Work out the finished part from the listing and answer in its coordinate system (mm). A direction names the side the tool comes from. Round coordinates to 2 decimals unless told otherwise and drop trailing zeros. Order: outer loops, then holes, each group sorted by start corner. A loop starts at its lowest first (then second) coordinate and runs counter-clockwise, first axis right, second up. Notation, with made-up numbers: M 14,-5.5 L 56,-5.5 A7 ccw 56,3.5 Z; hole C 19.5,74 d10. An arc over 180 degrees is marked long. Return JSON: item names as keys, results as strings.
from build123d import *

# Parameters (mm, degrees)
SKETCH1_W             = 66.04
SKETCH1_H             = 33.02
BOSS_EXTRUDE1_DEPTH   = 4.2418
FILLET1_R             = 1.27
SKETCH2_W             = 106.172
SKETCH2_H             = 36.322
BOSS_EXTRUDE2_DEPTH   = 6.604
F_3_CLEARANCE_HOLE1_D = 2.794
SKETCH6_W             = 69.85
SKETCH6_H             = 22.606
BOSS_EXTRUDE3_DEPTH   = 22.0472


with BuildPart() as part:
    # Sketch1 → Boss-Extrude1 (new body)
    with BuildSketch(Plane(origin=(0, 0, 0), x_dir=(1, 0, 0), z_dir=(0, 1, 0))):
        Rectangle(SKETCH1_W, SKETCH1_H)
    extrude(amount=BOSS_EXTRUDE1_DEPTH)

    # Fillet1
    fillet1_edges = [part.edges().sort_by_distance(p)[0] for p in [
        (33.02, 2.1209, 16.51),
        (-33.02, 2.1209, 16.51),
        (-33.02, 2.1209, -16.51),
        (33.02, 2.1209, -16.51),
    ]]
    fillet(fillet1_edges, radius=FILLET1_R)

    # Sketch2 → Boss-Extrude2 (add)
    with BuildSketch(Plane.XZ):
        Rectangle(SKETCH2_W, SKETCH2_H)
    extrude(amount=BOSS_EXTRUDE2_DEPTH)

    # #3 Clearance Hole1 (through all)
    with Locations(Plane(origin=(0, 0, 0), x_dir=(1, 0, 0), z_dir=(0, 1, 0))):
        with Locations((-48.3997, 0), (48.3997, 0)):
            Hole(F_3_CLEARANCE_HOLE1_D / 2)

    # Sketch6 → Boss-Extrude3 (add)
    with BuildSketch(Plane.XZ.offset(6.604)):
        Rectangle(SKETCH6_W, SKETCH6_H)
    extrude(amount=BOSS_EXTRUDE3_DEPTH)


solid = part.part
Item 1: Which of the six approach directions +Z, -Z, +X, -X, +Y, -Y give full straight-line access (tool end or side, diameter ignored) to faces 1 (the flat face through (-34.925, -17, 0)), 2 (the flat face through (-33.02, 2, 0)), 3 (the flat face through (33.02, 2, 0)), 4 (the flat face through (0, 2, 16.51)), 5 (the flat face through (0, -17, 11.303))?
Output:
{"face 1": "+Z, -Z, -X, -Y", "face 2": "+Z, -Z, -X, +Y", "face 3": "+Z, -Z, +X, +Y", "face 4": "+Z, +X, -X, +Y", "face 5": "+Z, +X, -X, -Y"}
Item 2: Find section C-C (y = -17.5). Determine the outline of the cut face in (x, z) (3 decimals).
Output:
{"outline": "M -34.925,-11.303 L 34.925,-11.303 L 34.925,11.303 L -34.925,11.303 Z"}
Item 3: Each of these flat-tipped pins is pushed along its axis until it touches: pin 1 (2.5 mm diameter, centred on x = 48.4, z = 0, fed in from +Y); pin 2 (11 mm diameter, centred on y = -20, z = 3, fed in from -X) (3 decimals); pin 3 (4 mm diameter, centred on x = 4, y = -24, fed in from -Z); pin 4 (1.3 mm diameter, centred on y = 2.5, z = -6.5, fed in from +X). Where does it stop, or does it pass through?
Output:
{"pin 1": "passes through", "pin 2": "stops at x = -34.925", "pin 3": "stops at z = -11.3", "pin 4": "stops at x = 33.02"}
Item 4: Consider line 1 along Z through (x, y) = (11, -22.5); line 2 along Y through (x, z) = (26, -12); line 3 along X through (y, z) = (-21, 9) (3 decimals). Determine where each line is inside the solid, lowest interval first. Write a range as [from, to].
Output:
{"line 1": "z = [-11.3, 11.3]", "line 2": "y = [-6.6, 4.24]", "line 3": "x = [-34.925, 34.925]"}
Item 5: Find section D-D (z = -9). Determine the outline of the cut face in (x, y) (3 decimals).
Output:
{"outline": "M -53.086,-6.604 L -34.925,-6.604 L -34.925,-28.651 L 34.925,-28.651 L 34.925,-6.604 L 53.086,-6.604 L 53.086,0 L 33.02,0 L 33.02,4.242 L -33.02,4.242 L -33.02,0 L -53.086,0 Z"}
Item 6: Find section A-A (z = 0). Determine the outline of the cut face in (x, y) (3 decimals), plus the area to 3 significant figures.
Output:
{"outline": "M -53.086,-6.604 L -49.797,-6.604 L -49.797,0 L -53.086,0 Z; M -47.003,-6.604 L -34.925,-6.604 L -34.925,-28.651 L 34.925,-28.651 L 34.925,-6.604 L 47.003,-6.604 L 47.003,0 L 33.02,0 L 33.02,4.242 L -33.02,4.242 L -33.02,0 L -47.003,0 Z; M 49.797,-6.604 L 53.086,-6.604 L 53.086,0 L 49.797,0 Z", "area": "2,480 mm^2"}
Item 7: The mould has two halves that part along X. Classify faces 6 (the flat face through (34.925, -17, 0)), 7 (the flat face through (0, -17, -11.303)), 8 (the cylindrical face through (-49.69, -3.35, 0.54)): pulls with the +X half, pulls with the -X half, needs draft (parallel to the pull), parting line crosses it, or undercut.
Output:
{"face 6": "pulls with the +X half", "face 7": "needs draft", "face 8": "undercut"}
Item 8: Find section B-B (z = 13). Determine the outline of the cut face in (x, y), plus the area to 3 significant figures.
Output:
{"outline": "M -53.09,-6.6 L 53.09,-6.6 L 53.09,0 L 33.02,0 L 33.02,4.24 L -33.02,4.24 L -33.02,0 L -53.09,0 Z", "area": "981 mm^2"}
